Source: CAD feature listing. Evaluate the final solid. Frame: model axes, mm. Give positions to 0.01 mm unless a question says otherwise; leave off trailing zeros. Order: outer loops, then holes, each group sorted by start corner. A loop starts at its lowest first (then second) coordinate and runs counter-clockwise, first axis right, second up.
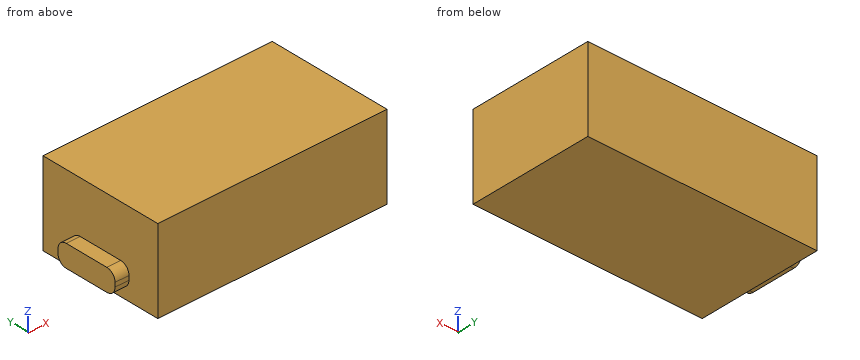
```python
from build123d import *

# Parameters (mm, degrees)
SKETCH_1_W      = 33
SKETCH_1_H      = 18
EXTRUDE_1_DEPTH = 12
EXTRUDE_2_DEPTH = 2


with BuildPart() as part:
    # Эскиз1 → Бобышка-Вытянуть1 (new body)
    with BuildSketch(Plane.XY):
        with Locations((16.5, 9)):
            Rectangle(SKETCH_1_W, SKETCH_1_H)
    extrude(amount=EXTRUDE_1_DEPTH)

    # Эскиз2 → Бобышка-Вытянуть2 (add)
    with BuildSketch(Plane.ZY):
        with BuildLine():
            Line((2.7, 4.53), (3.3, 4.53))
            ThreePointArc((3.3, 4.53), (4.20509668, 4.90490332), (4.58, 5.81))
            Line((4.58, 5.81), (4.58, 12.19))
            ThreePointArc((4.58, 12.19), (4.20509668, 13.09509668), (3.3, 13.47))
            Line((3.3, 13.47), (2.7, 13.47))
            ThreePointArc((2.7, 13.47), (1.79490332, 13.09509668), (1.42, 12.19))
            Line((1.42, 12.19), (1.42, 5.81))
            ThreePointArc((1.42, 5.81), (1.79490332, 4.90490332), (2.7, 4.53))
        make_face()
    extrude(amount=EXTRUDE_2_DEPTH)


solid = part.part
```
1) Section query D-D, the plane y = 3. Return the cut outline in (x, z).
Report:
outline: (0, 0) - (33, 0) - (33, 12) - (0, 12) - close
2) Section query C-C, the plane y = 12.75. Return the cut outline in (x, z), and give its area (3 significant figures).
Report:
outline: (-2, 1.55) - (0, 1.55) - (0, 0) - (33, 0) - (33, 12) - (0, 12) - (0, 4.45) - (-2, 4.45) - close
area: 402 mm2
3) Pin query (flat end, axial travel): pin 1 (1 mm diameter, centred on x = -1, y = 9.5, fed in from +Z); pin 2 (0.5 mm diameter, centred on x = -0.5, z = 3, fed in from +Y). Return the tip coordinate at first contact, or that it passes through.
Report:
pin 1: stops at z = 4.58
pin 2: stops at y = 13.47
4) Section query A-A, the plane y = 6.5. Return the cut outline in (x, z), and give its area (3 significant figures).
Report:
outline: (-2, 1.42) - (0, 1.42) - (0, 0) - (33, 0) - (33, 12) - (0, 12) - (0, 4.58) - (-2, 4.58) - close
area: 402 mm2
5) Section query B-B, the plane z = 9.5. Return the cut outline in (x, y), and give its area (3 significant figures).
Report:
outline: (0, 0) - (33, 0) - (33, 18) - (0, 18) - close
area: 594 mm2
6) Material intervals for L1, parallel to X at y = 15, z = 5, sorted ascending.
Report:
L1: x = 0 to 33
